Design review of the part shown in the three views and the two pictorial views. Dimensions are in mm from the part's minimum x, y and z. A direction names the side the tool comes from. Give positions to 0.01 mm unless a question says otherwise; leave off trailing zeros. Write each loop counter-clockwise with the first axis right and the second up, starting at its lowest first coordinate (ties: lowest second). Pieces come first, ordered by that corner, then holes.
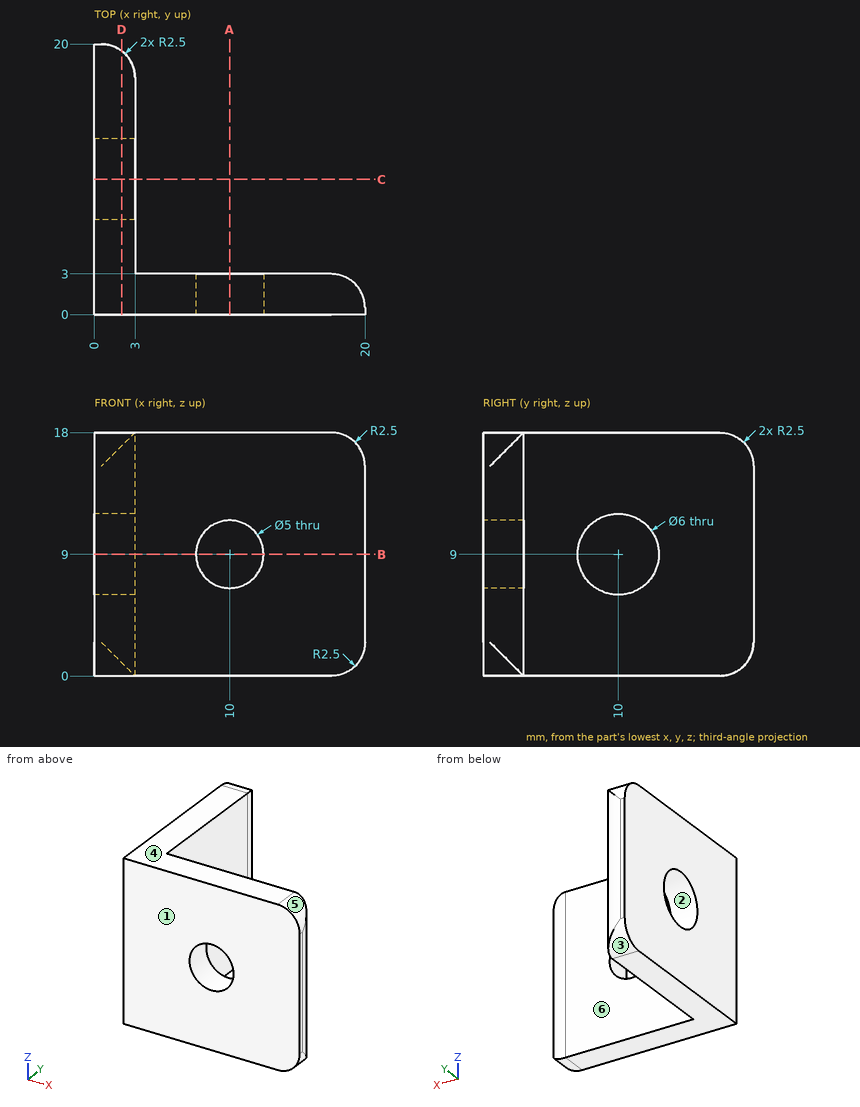
(1) Clearance check with a flat-ended pin moving along its axis: P1, Ø7, axis at x = 10.5, z = 13.5, coming from the +Y side. State where the tip first meets the part, or that it passes through.
Resolved:
P1: stops at y = 3
(2) Consider section B-B, the plane z = 9. Give the boundary of the cut face in (x, y).
Resolved:
outline: (0, 0) - (7.5, 0) - (7.5, 3) - (3, 3) - (3, 7) - (0, 7) - close; (0, 13) - (3, 13) - (3, 17.5) arc R2.5 ccw to (0.5, 20) - (0, 20) - close; (12.5, 0) - (20, 0) - (20, 0.5) arc R2.5 ccw to (17.5, 3) - (12.5, 3) - close
(3) Consider section D-D, the plane x = 2. Give the boundary of the cut face in (y, z), then the cut area to 3 significant figures.
Resolved:
outline: (0, 0) - (17.5, 0) arc R2.5 ccw to (19.5, 1) - (19.5, 17) arc R2.5 ccw to (17.5, 18) - (0, 18) - close; hole circle Ø6 at (10, 9)
area: 322 mm2
(4) Mouldability with a two-part tool opening along Y and no side actions: class the marked faces 1, 2, 3 and 4 as pulls with the +Y half, pulls with the -Y half, needs draft (parallel to the pull), parting line crosses it, or undercut.
Resolved:
face 1: pulls with the -Y half
face 2: undercut
face 3: pulls with the +Y half
face 4: needs draft
(5) Tool access review of the marked faces 5 and 6: name each direction out of +Z, -Z, +X, -X, +Y, -Y from which nothing blocks a thin tool from reaching the whole face with its end or side.
Resolved:
face 5: +Z, +X, +Y, -Y
face 6: +Z, -Z, +X, +Y
(6) Consider section A-A, the plane x = 10. Give the boundary of the cut face in (y, z).
Resolved:
outline: (0, 0) - (3, 0) - (3, 6.5) - (0, 6.5) - close; (0, 11.5) - (3, 11.5) - (3, 18) - (0, 18) - close
(7) Consider section C-C, the plane y = 10. Give the boundary of the cut face in (x, z).
Resolved:
outline: (0, 0) - (3, 0) - (3, 6) - (0, 6) - close; (0, 12) - (3, 12) - (3, 18) - (0, 18) - close
(8) To check wall thickness, follow L1, parallel to Z at x = 0.8, y = 10; L2, parallel to Z at x = 10, y = 1.9; L3, parallel to Y at x = 5, z = 5.75. State the ranges of each line that lie inside material, in increasing order.
Resolved:
L1: z = 0 to 6, 12 to 18
L2: z = 0 to 6.5, 11.5 to 18
L3: y = 0 to 3
